from build123d import *

# Parameters (mm, degrees)
PAD_DEPTH             = 2
SKETCH001_R           = 2.5
PAD001_DEPTH          = 6
SKETCH002_R           = 1.25
POCKET_DEPTH          = 8
POLARPATTERN_COUNT    = 8
POLARPATTERN001_COUNT = 8


with BuildPart() as part:
    # Sketch → Pad (new body)
    with BuildSketch(Plane.XY):
        Polygon((24.944747, -10.332453), (24.944747, 10.332453), (10.332453, 24.944747), (-10.332453, 24.944747), (-24.944747, 10.332453), (-24.944747, -10.332453), (-10.332453, -24.944747), (10.332453, -24.944747), align=None)
    extrude(amount=PAD_DEPTH)

    # Sketch001 (on Face10 of Pad) → Pad001 (join)
    with BuildSketch(Plane.XY.offset(2)):
        with Locations((8.419036, 20.32535)):
            Circle(SKETCH001_R)
    pad001 = extrude(amount=PAD001_DEPTH)

    # Sketch002 (on Face12 of Pad001) → Pocket (cut)
    with BuildSketch(Plane.XY.offset(8)):
        with Locations((8.419036, 20.32535)):
            Circle(SKETCH002_R)
    pocket = extrude(amount=-POCKET_DEPTH, mode=Mode.SUBTRACT)

    # PolarPattern: Pad001 ×8 about axis
    polarpattern_axis = Axis((0, 0, 2), (0, 0, 1))
    for i in range(1, POLARPATTERN_COUNT):
        add(pad001.rotate(polarpattern_axis, i * 360 / POLARPATTERN_COUNT))

    # PolarPattern001: Pocket ×8 about axis
    polarpattern001_axis = Axis((0, 0, 8), (0, 0, 1))
    for i in range(1, POLARPATTERN001_COUNT):
        add(pocket.rotate(polarpattern001_axis, i * 360 / POLARPATTERN001_COUNT), mode=Mode.SUBTRACT)


solid = part.part
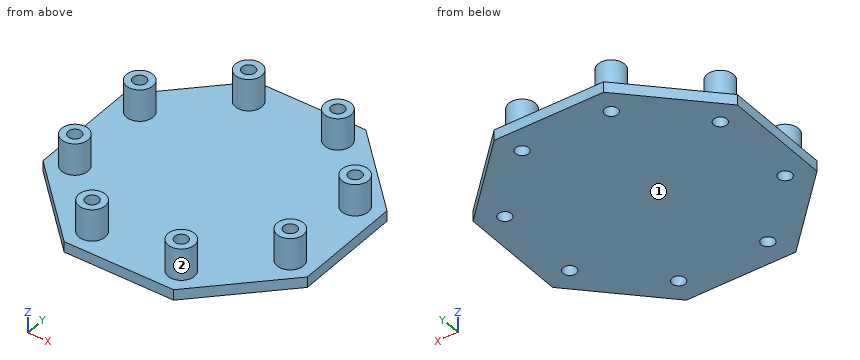
Check sheet for the modelled part. Datum: model origin and axes. Units: mm. Face numbers are marked on the shaded views. Give positions to 0.01 mm unless a question says otherwise; leave off trailing zeros. Write each loop counter-clockwise with the first axis right and the second up, starting at its lowest first coordinate (ties: lowest second). Pieces come first, ordered by that corner, then holes. Notation, with made-up numbers: (-13.5, 1.5) -> (7.5, 1.5) arc R35 ccw to (7.5, 34.5) -> close; hole circle Ø1 at (-11, 79.5). An arc over 180 degrees is marked (long way). Write item = value, one per line.
Item 1: Release check for a two-part mould opening along X. For the marked faces 1 and 2 record: +X half, -X half, draft (parallel to the pull), parting line (faces both ways), or undercut.
Output:
face_1 = draft
face_2 = undercut
Item 2: Sectioned sample at C-C on z = 4.25. Count the separate pieces of the cut face and the enclosed holes in it, and give its area (3 significant figures).
Output:
separate_pieces = 8
enclosed_holes = 8
area = 118 mm^2
Item 3: Sectioned sample at A-A on x = -9. Record the boundary of the cut face in (y, z).
Output:
outline = (-24.94, 0) -> (-21.43, 0) -> (-21.43, 8) -> (-22.76, 8) -> (-22.76, 2) -> (-24.94, 2) -> close; (-19.22, 0) -> (19.22, 0) -> (19.22, 8) -> (17.89, 8) -> (17.89, 2) -> (-17.89, 2) -> (-17.89, 8) -> (-19.22, 8) -> close; (21.43, 0) -> (24.94, 0) -> (24.94, 2) -> (22.76, 2) -> (22.76, 8) -> (21.43, 8) -> close
Item 4: Scan lines: probe 1 along X at (y, z) = (-20.5, 4.75); probe 2 along Y at (x, z) = (8, 5.5); probe 3 along Y at (x, z) = (-7.5, 3). Record each from-to range of solid material in increasing order. Write a range as from..to.
Output:
probe_1 = -10.91..-9.66, -7.18..-5.93, 5.93..7.18, 9.66..10.91
probe_2 = -22.79..-21.5, -19.15..-17.86, 17.86..19.15, 21.5..22.79
probe_3 = -22.65..-21.17, -19.48..-18, 18..19.48, 21.17..22.65
Item 5: Gauge pin test, flat ends, axial feed: pin 1 (4 mm diameter, centred on x = -16.5, y = 18, fed in from +Z); pin 2 (4 mm diameter, centred on y = 8.5, z = 5, fed in from -X). Record the tip position at first contact, or that the pin passes through.
Output:
pin_1 = 2
pin_2 = -22.83
